Design review of the part built by this model. Coordinates are the model's own, in mm. Face numbers are marked on the shaded views. A direction names the side the tool comes from. Coordinates: 2 decimals unless noted, no trailing zeros. Loops run counter-clockwise (first coordinate to the right, second up) from the corner with the lowest first, then second, coordinate; pieces in that order, holes last.
Q1. Wall thickness on probe 1 along X at (y, z) = (-29, 7); probe 2 along Y at (x, z) = (50, 2); probe 3 along X at (y, z) = (-15, -40): over which ranges is each line inside the solid? List them lowest first.
Q2. Add section B-B on y = -37. Give the boundary of the cut face in (x, z), and give its area (3 significant figures).
Q3. Draft analysis for pull direction X (two halves, no side actions). For the marked faces 3, 4 and 5, state which applies: released by +X, released by -X, zero draft, split by the parting line, or undercut.
Q4. Add section A-A on z = -25. Give the boundary of the cut face in (x, y), and give its area (3 significant figures).
Q5. Machinability: for the marked faces 1 and 2, which of the approach directions +Z, -Z, +X, -X, +Y, -Y give a long, thin tool a straight path to every point of the face, cutting with its end or side? Answer none if there is none.
Q6. For P1, Ø20, axis at x = -14.5, y = 17.5, coming from the -Z side, flat-tipped, find the tip position at first contact; note if it passes through.
```python
from build123d import *

# Parameters (mm, degrees)
SKETCH1_W           = 127
SKETCH1_H           = 76.2
SKETCH1_R           = 2.978797174
SKETCH1_R_2         = 3
SKETCH1_W_2         = 60
SKETCH1_H_2         = 20
SKETCH1_W_3         = 13
SKETCH1_H_3         = 13
BOSS_EXTRUDE1_DEPTH = 8.89
SKETCH3_W           = 127
SKETCH3_H           = 76.2
SKETCH3_R           = 5.518797174
SKETCH3_W_2         = 18.08
SKETCH3_H_2         = 18.08
SKETCH3_R_2         = 3
SKETCH3_W_3         = 65.08
SKETCH3_H_3         = 25.08
CUT_EXTRUDE1_DEPTH  = 3.81
BOSS_EXTRUDE2_START = -5.08
SKETCH5_W           = 129.54
SKETCH5_H           = 78.74
SKETCH5_W_2         = 127
SKETCH5_H_2         = 76.2
BOSS_EXTRUDE2_DEPTH = 5.08
SKETCH6_W           = 139.7
SKETCH6_H           = 88.9
SKETCH6_W_2         = 129.54
SKETCH6_H_2         = 78.74
BOSS_EXTRUDE3_DEPTH = 76.2
CUT_EXTRUDE3_REACH  = 141.7
SKETCH7_W           = 6.952697557
SKETCH7_H           = 10.320960494


with BuildPart() as part:
    # Sketch1 → Boss-Extrude1 (new body)
    with BuildSketch(Plane.XY):
        Rectangle(SKETCH1_W, SKETCH1_H)
        with Locations((-12.7, -16.51)):
            Circle(SKETCH1_R, mode=Mode.SUBTRACT)
        with Locations((12.7, -16.51)):
            Circle(SKETCH1_R, mode=Mode.SUBTRACT)
        with Locations((-15.875, -29.21)):
            Circle(SKETCH1_R_2, mode=Mode.SUBTRACT)
        with Locations((-9.525, -29.21)):
            Circle(SKETCH1_R_2, mode=Mode.SUBTRACT)
        with Locations((9.525, -29.21)):
            Circle(SKETCH1_R_2, mode=Mode.SUBTRACT)
        with Locations((15.875, -29.21)):
            Circle(SKETCH1_R_2, mode=Mode.SUBTRACT)
        with Locations((-50.124380999, -10.001211499)):
            Circle(SKETCH1_R_2, mode=Mode.SUBTRACT)
        with Locations((0, 21.75)):
            Rectangle(SKETCH1_W_2, SKETCH1_H_2, mode=Mode.SUBTRACT)
        with Locations((-45.39, 21.75)):
            Rectangle(SKETCH1_W_3, SKETCH1_H_3, mode=Mode.SUBTRACT)
        with Locations((45.39, 21.75)):
            Rectangle(SKETCH1_W_3, SKETCH1_H_3, mode=Mode.SUBTRACT)
        with Locations((-45.39, -22.996165479)):
            Rectangle(SKETCH1_W_3, SKETCH1_H_3, mode=Mode.SUBTRACT)
    extrude(amount=BOSS_EXTRUDE1_DEPTH)

    # Sketch3 → Cut-Extrude1 (cut)
    with BuildSketch(Plane(origin=(0, 0, 0), x_dir=(-1, 0, 0), z_dir=(0, 0, -1))):
        Rectangle(SKETCH3_W, SKETCH3_H)
        with BuildLine():
            ThreePointArc((-12.7, -24.670068833), (-6.965498095, -24.296696631), (-3.985, -29.21))
            ThreePointArc((-3.985, -29.21), (-6.965498095, -34.123303369), (-12.7, -33.749931167))
            ThreePointArc((-12.7, -33.749931167), (-21.415, -29.21), (-12.7, -24.670068833))
        make_face(mode=Mode.SUBTRACT)
        with Locations((-12.7, -16.51)):
            Circle(SKETCH3_R, mode=Mode.SUBTRACT)
        with BuildLine():
            ThreePointArc((12.7, -24.670068833), (18.434501905, -24.296696631), (21.415, -29.21))
            ThreePointArc((21.415, -29.21), (18.434501905, -34.123303369), (12.7, -33.749931167))
            ThreePointArc((12.7, -33.749931167), (3.985, -29.21), (12.7, -24.670068833))
        make_face(mode=Mode.SUBTRACT)
        with Locations((45.39, -22.996165479)):
            Rectangle(SKETCH3_W_2, SKETCH3_H_2, mode=Mode.SUBTRACT)
        with Locations((12.7, -16.51)):
            Circle(SKETCH3_R, mode=Mode.SUBTRACT)
        with Locations((50.124380999, -10.001211499)):
            Circle(SKETCH3_R_2, mode=Mode.SUBTRACT)
        with Locations((-45.39, 21.75)):
            Rectangle(SKETCH3_W_2, SKETCH3_H_2, mode=Mode.SUBTRACT)
        with Locations((0, 21.75)):
            Rectangle(SKETCH3_W_3, SKETCH3_H_3, mode=Mode.SUBTRACT)
        with Locations((45.39, 21.75)):
            Rectangle(SKETCH3_W_2, SKETCH3_H_2, mode=Mode.SUBTRACT)
    extrude(amount=-CUT_EXTRUDE1_DEPTH, mode=Mode.SUBTRACT)

    # Sketch5 → Boss-Extrude2 (add)
    with BuildSketch(Plane.XY.offset(8.89).offset(BOSS_EXTRUDE2_START)):
        Rectangle(SKETCH5_W, SKETCH5_H)
        Rectangle(SKETCH5_W_2, SKETCH5_H_2, mode=Mode.SUBTRACT)
    extrude(amount=BOSS_EXTRUDE2_DEPTH)

    # Sketch6 → Boss-Extrude3 (add)
    with BuildSketch(Plane.XY.offset(8.89)):
        Rectangle(SKETCH6_W, SKETCH6_H)
        Rectangle(SKETCH6_W_2, SKETCH6_H_2, mode=Mode.SUBTRACT)
    extrude(amount=-BOSS_EXTRUDE3_DEPTH)

    # Sketch7 → Cut-Extrude3 (cut, up to next)
    with BuildSketch(Plane.ZY.offset(69.85), mode=Mode.PRIVATE) as cut_extrude3_sk1:
        with Locations((0.333651222, 1.522792989)):
            Rectangle(SKETCH7_W, SKETCH7_H)
    cut_extrude3_tool1 = extrude(cut_extrude3_sk1.sketch, amount=-CUT_EXTRUDE3_REACH, mode=Mode.PRIVATE) & part.part
    add(cut_extrude3_tool1.solids().sort_by_distance((-69.85, 1.522793, 0.333651))[0], mode=Mode.SUBTRACT)


solid = part.part
```
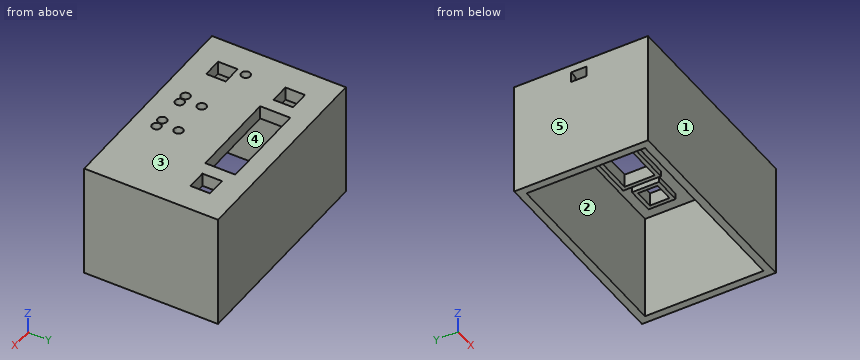
Entries:
1. probe 1: x = -69.85 to -51.89, -38.89 to -18.87, -12.88 to -12.52, -6.53 to 6.53, 12.52 to 12.88, 18.87 to 69.85
1. probe 2: y = -44.45 to -39.37, 12.71 to 15.25, 28.25 to 30.79, 39.37 to 44.45
1. probe 3: x = -69.85 to -64.77, 64.77 to 69.85
2. outline: (-69.85, -67.31) - (-64.77, -67.31) - (-64.77, 3.81) - (64.77, 3.81) - (64.77, -67.31) - (69.85, -67.31) - (69.85, 8.89) - (-69.85, 8.89) - close
2. area: 1,430 mm2
3. face 3: zero draft
3. face 4: undercut
3. face 5: released by -X
4. outline: (-69.85, -44.45) - (69.85, -44.45) - (69.85, 44.45) - (-69.85, 44.45) - close; hole (-64.77, -39.37) - (64.77, -39.37) - (64.77, 39.37) - (-64.77, 39.37) - close
4. area: 2,220 mm2
5. face 1: +Z, -Z, +X, -X, -Y
5. face 2: -Z
6. P1: stops at z = 0
